Check sheet for the modelled part. Datum: model origin and axes. Units: mm. Coordinates: 2 decimals unless noted, no trailing zeros. Write each loop counter-clockwise with the first axis right and the second up, starting at its lowest first coordinate (ties: lowest second). Pieces come first, ordered by that corner, then holes. Notation, with made-up numbers: (66, 51.25) - (84, 51.25) arc R20 cw to (84, 61.25) - close; hole circle Ø5 at (23, 33). An arc over 180 degrees is marked (long way). Use one line per item in the form item = value. Start each with the question number.
1. Scan lines: line 1 along Z through (x, y) = (-47.5, 1.25); line 2 along Z through (x, y) = (-16.5, 1.8). Record each from-to range of solid material in increasing order.
2. Cross-section at B-B on y = 2.1. Record the boundary of the cut face in (x, z).
3. Cross-section at A-A on z = -44.5. Record the boundary of the cut face in (x, y).
4. Cross-section at C-C on x = -32.5. Record the boundary of the cut face in (y, z).
5. Cross-section at D-D on z = 11. Record the boundary of the cut face in (x, y).
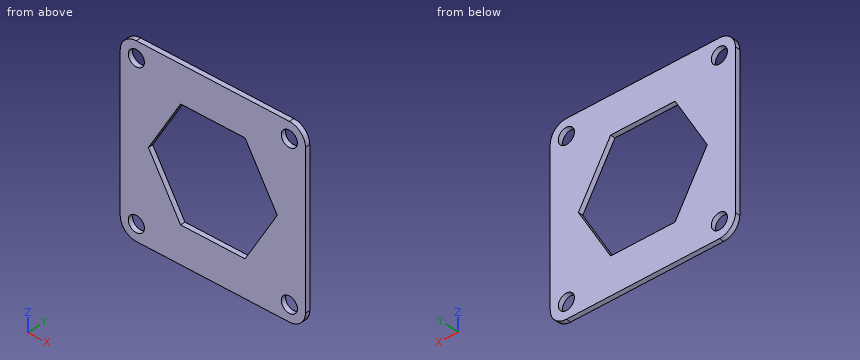
Autodesk Fusion 360 part; units mm, degrees
sketch "Sketch1" plane through (0, 0, 0) normal (0, 1, 0) x (1, 0, 0)
  line L0 (47.5, -57.5) -> (-47.5, -57.5)
  line L1 (-57.5, -47.5) -> (-57.5, 47.5)
  line L2 (-47.5, 57.5) -> (47.5, 57.5)
  line L3 (57.5, 47.5) -> (57.5, -47.5)
  line L4 (57.5, -57.5) -> (-57.5, 57.5) construction
  line L5 (-57.5, -57.5) -> (57.5, 57.5) construction
  arc A0 (57.5, 47.5) -> (47.5, 57.5) centre (47.5, 47.5) ccw
  arc A1 (47.5, -57.5) -> (57.5, -47.5) centre (47.5, -47.5) ccw
  arc A2 (-57.5, -47.5) -> (-47.5, -57.5) centre (-47.5, -47.5) ccw
  arc A3 (-47.5, 57.5) -> (-57.5, 47.5) centre (-47.5, 47.5) ccw
  circle A4 centre (-47.5, 47.5) radius 5
  circle A5 centre (47.5, 47.5) radius 5
  circle A6 centre (47.5, -47.5) radius 5
  circle A7 centre (-47.5, -47.5) radius 5
  line L6 (40, 0) -> (20, 34.641)
  line L7 (20, 34.641) -> (-20, 34.641)
  line L8 (-20, 34.641) -> (-40, 0)
  line L9 (-40, 0) -> (-20, -34.641)
  line L10 (-20, -34.641) -> (20, -34.641)
  line L11 (20, -34.641) -> (40, 0)
  dimension "d1" = 115
  dimension "d2" = 115
  dimension "d3" = 10
  dimension "d4" = 10
  dimension "d5" = 10
  dimension "d6" = 10
  dimension "d7" = 10
  dimension "d8" = 10
  dimension "d9" = 40
extrude "Extrude1" add sketch "Sketch1" along normal blind 3
Final values:
q1.line_1 = -57.5 to -52.5, -42.5 to 42.5, 52.5 to 57.5
q1.line_2 = -57.5 to -34.64, 34.64 to 57.5
q2.outline = (-57.5, -47.5) arc R10 ccw to (-47.5, -57.5) - (47.5, -57.5) arc R10 ccw to (57.5, -47.5) - (57.5, 47.5) arc R10 ccw to (47.5, 57.5) - (-47.5, 57.5) arc R10 ccw to (-57.5, 47.5) - close; hole circle Ø10 at (-47.5, -47.5); hole circle Ø10 at (-47.5, 47.5); hole (-40, 0) - (-20, -34.64) - (20, -34.64) - (40, 0) - (20, 34.64) - (-20, 34.64) - close; hole circle Ø10 at (47.5, -47.5); hole circle Ø10 at (47.5, 47.5)
q3.outline = (-57.5, 0) - (-51.5, 0) - (-51.5, 3) - (-57.5, 3) - close; (-43.5, 0) - (43.5, 0) - (43.5, 3) - (-43.5, 3) - close; (51.5, 0) - (57.5, 0) - (57.5, 3) - (51.5, 3) - close
q4.outline = (0, -57.5) - (3, -57.5) - (3, -12.99) - (0, -12.99) - close; (0, 12.99) - (3, 12.99) - (3, 57.5) - (0, 57.5) - close
q5.outline = (-57.5, 0) - (-33.65, 0) - (-33.65, 3) - (-57.5, 3) - close; (33.65, 0) - (57.5, 0) - (57.5, 3) - (33.65, 3) - close
